Verification items for this drawing (mm, ordinates from the low corner). Give positions to 0.01 mm unless a question says otherwise; leave off trailing zeros. Order: outer loops, then holes, each group sorted by start corner. A loop starts at its lowest first (then second) coordinate and runs counter-clockwise, first axis right, second up. Notation, with made-up numbers: M 52,37 L 61,37 A20 cw 61,75 Z; hole C 71,58.5 d3. An arc over 180 degrees is marked long. Return JSON: item names as keys, results as strings. Group by question number.
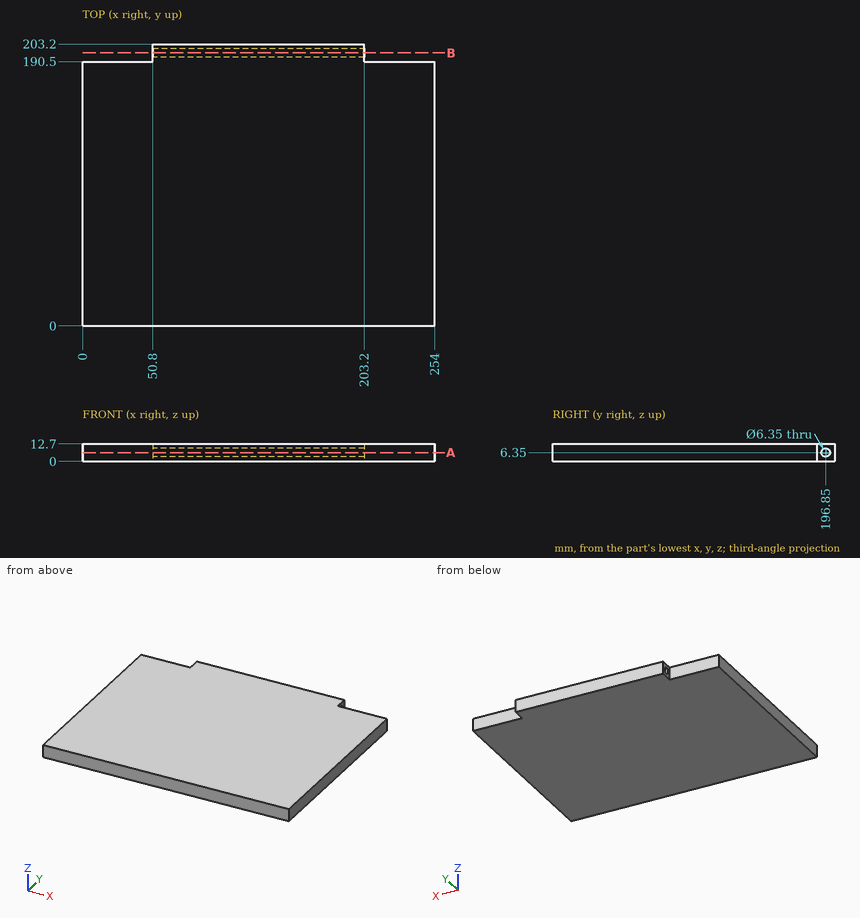
1) Material ranges on line 1 along Y through (x, z) = (136, 6.35) (3 decimals); line 2 along Z through (x, y) = (164.5, 196.85) (3 decimals); line 3 along Y through (x, z) = (44, 9.25), recorded low to high.
2) Depth check by flat-ended pin: P1, Ø1, axis at x = 202, y = 89, coming from the -Z side; P2, Ø6.5, axis at x = 237.5, z = 7, coming from the +Y side; P3, Ø6.5, axis at y = 194, z = 9, coming from the +X side. Enter the tip coordinate at first touch or a pass-through.
3) Sectioned sample at A-A on z = 6.35. Record the boundary of the cut face in (x, y) (3 decimals), then the cut area to 3 significant figures.
4) Sectioned sample at B-B on y = 196.85. Record the boundary of the cut face in (x, z) (3 decimals).
Reply:
{
 "1": {"line 1": "0 to 193.675, 200.025 to 203.2", "line 2": "0 to 3.175, 9.525 to 12.7", "line 3": "0 to 190.5"},
 "2": {"P1": "z = 0", "P2": "y = 190.5", "P3": "x = 203.2"},
 "3": {"outline": "M 0,0 L 254,0 L 254,190.5 L 203.2,190.5 L 203.2,193.675 L 50.8,193.675 L 50.8,190.5 L 0,190.5 Z; M 50.8,200.025 L 203.2,200.025 L 203.2,203.2 L 50.8,203.2 Z", "area": "49,400 mm^2"},
 "4": {"outline": "M 50.8,0 L 203.2,0 L 203.2,3.175 L 50.8,3.175 Z; M 50.8,9.525 L 203.2,9.525 L 203.2,12.7 L 50.8,12.7 Z"}
}
